Part model, mm, in its own coordinate system. A direction names the side the tool comes from. Round coordinates to 2 decimals unless told otherwise and drop trailing zeros. Order: outer loops, then holes, each group sorted by start corner. A loop starts at its lowest first (then second) coordinate and runs counter-clockwise, first axis right, second up. Notation, with made-up numbers: M 25.25,-10.5 L 82.25,-10.5 A10 cw 82.25,8.5 Z; hole C 23,47.25 d7. An arc over 180 degrees is marked long. One line per question, with ' | ' between items.
from build123d import *

# Parameters (mm, degrees)
F1_DEPTH = 15
F3_DEPTH = 130
F5_DEPTH = 15


with BuildPart() as f1:
    # F0 (on Top) → F1 (new body)
    with BuildSketch(Plane.XY):
        Polygon((171.201938, 23.315855), (0, 0), (0, -150), (246.201938, -106.587956), align=None)
        Polygon((0, -150), (0, 0), (-171.201938, 23.315855), (-246.201938, -106.587956), align=None)
    extrude(amount=F1_DEPTH)

    # F2 (on face) → F3 (join)
    with BuildSketch(Plane.XY.offset(15)):
        Polygon((-171.201938, 23.315855), (-246.201938, -106.587956), (-231.429822, -109.192678), (-163.82086, 8.290785), (0, -14.019847), (163.82086, 8.290785), (231.429822, -109.192678), (246.201938, -106.587956), (171.201938, 23.315855), (156.339139, 21.291702), (0, 0), (-156.339139, 21.291702), align=None)
    extrude(amount=F3_DEPTH)

    # F4 (on face) → F5 (join)
    with BuildSketch(Plane.XY.offset(145)):
        Polygon((-171.201938, 23.315855), (-246.201938, -106.587956), (0, -150), (246.201938, -106.587956), (171.201938, 23.315855), (0, 0), align=None)
    extrude(amount=F5_DEPTH)


solid = f1.part
1) Probe line 1 (Z direction, x = -129.5, y = -70); line 2 (X direction, y = -25, z = 82.5); line 3 (X direction, y = -97.5, z = 76) (3 decimals). List the from-to ranges inside material, lowest first. Write a range as [from, to].
The answers:
line 1: z = [0, 15], [145, 160] | line 2: x = [-199.1, -182.98], [182.98, 199.1] | line 3: x = [-240.955, -224.701], [224.701, 240.955]
2) Saw through at B-B (x = 119.5). List the corners of the cut face in (y, z), plus the area to 3 significant figures.
The answers:
outline: M -128.93,0 L 16.27,0 L 16.27,160 L -128.93,160 L -128.93,145 L 2.25,145 L 2.25,15 L -128.93,15 Z | area: 6,180 mm²
3) Saw through at C-C (z = 100.5). List the corners of the cut face in (x, y).
The answers:
outline: M -246.2,-106.59 L -231.43,-109.19 L -163.82,8.29 L 0,-14.02 L 163.82,8.29 L 231.43,-109.19 L 246.2,-106.59 L 171.2,23.32 L 0,0 L -171.2,23.32 Z
4) Saw through at D-D (y = -100). List the corners of the cut face in (x, z).
The answers:
outline: M -242.4,0 L 242.4,0 L 242.4,160 L -242.4,160 Z; hole M -226.14,15 L 226.14,15 L 226.14,145 L -226.14,145 Z
5) Two-plate mould, pull along Z, no slides. Class faces 1 (the face through (-198.099, -51.273, 79.09)), 2 (the face through (121.378, -128.598, 152.395)), 3 (the face through (80.76, -3.02, 79.09)), 4 (the face through (-3, -62, 160)): released by +Z, released by -Z, zero draft, split by the parting line, or undercut.
The answers:
face 1: undercut | face 2: zero draft | face 3: undercut | face 4: released by +Z
6) Which spindle directions (+Z, -Z, +X, -X, +Y, -Y) get a long thin tool onto all of the face, cutting with end or side? Do faces 5 (the face through (-124.82, -127.99, 152.4)), 6 (the face through (197.152, -49.629, 79.09)). Say none if no direction does.
The answers:
face 5: +Z, -Z, -X, -Y | face 6: -Y
7) Saw through at A-A (y = -61). List the corners of the cut face in (x, z).
The answers:
outline: M -219.88,0 L 219.88,0 L 219.88,160 L -219.88,160 Z; hole M -203.7,15 L 203.7,15 L 203.7,145 L -203.7,145 Z
8) Drop flat-ended pins along their axis: pin 1 (10 mm diameter, centred on y = -19.5, z = 31, fed in from +X); pin 2 (3 mm diameter, centred on x = -38, z = 62, fed in from +Y); pin 3 (8 mm diameter, centred on x = 146.5, z = 89, fed in from -Y). Give the stop position or say it passes through.
The answers:
pin 1: stops at x = 198.81 | pin 2: stops at y = 5.38 | pin 3: stops at y = 5.39
